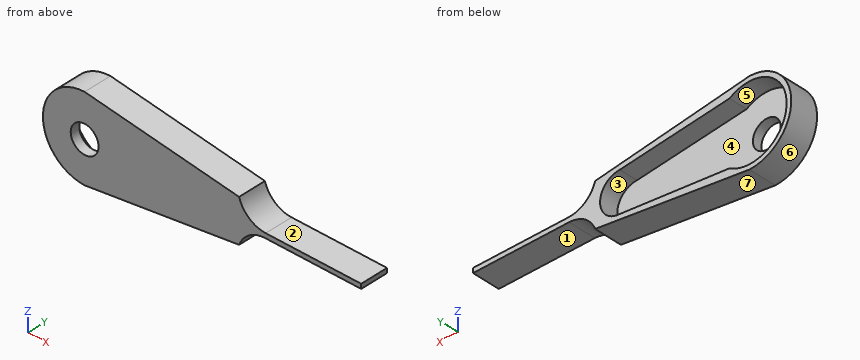
```python
from build123d import *

# Parameters (mm, degrees)
SKETCH2_R           = 1.5
BOSS_EXTRUDE1_DEPTH = 1
BOSS_EXTRUDE2_DEPTH = 3
FILLET1_R           = 3
FILLET2_R           = 3


with BuildPart() as part:
    # Sketch2 → Boss-Extrude1 (new body)
    with BuildSketch(Plane(origin=(0, 0, 0), x_dir=(1, 0, 0), z_dir=(0, 1, 0))):
        with BuildLine():
            Line((-12.939762178, 2.094266176), (-24.821781773, 3.29179515))
            ThreePointArc((-24.821781773, 3.29179515), (-30.987291256, -0.071668068), (-24.821747911, -3.435069212))
            Line((-24.821747911, -3.435069212), (-12.987160246, -2.166440487))
            ThreePointArc((-12.987160246, -2.166440487), (-10.8566751, -0.059524017), (-12.939762178, 2.094266176))
        make_face()
        with Locations(Location((-26.987114413, 0, 0), (0, 0, 270))):
            Circle(SKETCH2_R, mode=Mode.SUBTRACT)
    extrude(amount=BOSS_EXTRUDE1_DEPTH)

    # Sketch2<3> → Boss-Extrude2 (add)
    with BuildSketch(Plane(origin=(0, 0, 0), x_dir=(1, 0, 0), z_dir=(0, 1, 0))):
        with BuildLine():
            Line((-10.322349305, -2.339041202), (-10.322728968, -0.2))
            Line((-10.322728968, -0.2), (2.851540312, -0.2))
            Line((2.851540312, -0.2), (2.851540312, 0.3))
            Line((2.851540312, 0.3), (-10.322728968, 0.3))
            Line((-10.322728968, 0.3), (-10.322728968, 2.279037645))
            Line((-10.322728968, 2.279037645), (-26.987114411, 4.428185187))
            ThreePointArc((-26.987114411, 4.428185187), (-31.48694753, -0.071647931), (-26.987114411, -4.57148105))
            Line((-26.987114411, -4.57148105), (-10.322349305, -2.339041202))
        make_face()
        with BuildLine():
            ThreePointArc((-12.939762178, 2.094266176), (-10.8566751, -0.059524017), (-12.987160246, -2.166440487))
            Line((-12.987160246, -2.166440487), (-24.821747911, -3.435069212))
            ThreePointArc((-24.821747911, -3.435069212), (-30.987291256, -0.071668068), (-24.821781773, 3.29179515))
            Line((-24.821781773, 3.29179515), (-12.939762178, 2.094266176))
        make_face(mode=Mode.SUBTRACT)
    extrude(amount=BOSS_EXTRUDE2_DEPTH)

    # Fillet1
    # the kernel refuses this fillet: 3 mm, written as the material it adds along each edge
    with BuildSketch(Plane(origin=(-10.322728968, 0, -0.3), x_dir=(1, 0, 0), z_dir=(0, 1, 0))) as fillet1_piece_1:
        with BuildLine():
            CenterArc((2.820928193, 3), FILLET1_R, 199.896419226, 70.103580774)
            Line((0, 1.979037645), (-0.056418564, 1.958618398))
            ThreePointArc((-0.056418564, 1.958618398), (-0.06, 0.989518822), (-0.06, 0))
            Line((-0.06, 0), (0, -0.06))
            Line((0, -0.06), (2.820928193, -0.06))
            Line((2.820928193, -0.06), (2.820928193, 0))
        make_face()
    extrude(amount=3)

    # Fillet2
    # the kernel refuses this fillet: 3 mm, written as the material it adds along each edge
    with BuildSketch(Plane(origin=(-10.322728968, 0, 0.2), x_dir=(1, 0, 0), z_dir=(0, 1, 0))) as fillet2_piece_1:
        with BuildLine():
            CenterArc((2.874183753, -3), FILLET2_R, 90, 73.322386102)
            Line((0.000379663, -2.139041202), (-0.057096419, -2.121822026))
            ThreePointArc((-0.057096419, -2.121822026), (-0.059810168, -1.069531251), (-0.059999999, -1.065e-05))
            Line((-0.059999999, -1.065e-05), (0, 0.06))
            Line((0, 0.06), (2.874183753, 0.06))
            Line((2.874183753, 0.06), (2.874183753, 0))
        make_face()
    extrude(amount=3)


solid = part.part
```
Read the model definition and answer for the solid it produces. Units are mm, in the model's axes. Face numbers are marked on the shaded views. A direction names the side the tool comes from. Give positions to 0.01 mm unless a question says otherwise; leave off trailing zeros. Loops run counter-clockwise (first coordinate to the right, second up) from the corner with the lowest first, then second, coordinate; pieces in that order, holes last.
Item 1: Find the intervals of material crossed by line 1 along X through (y, z) = (0.6, 0); line 2 along Z through (x, y) = (-4.5, 0.4); line 3 along Y through (x, z) = (-15, 0.25), in increasing order.
Item 2: The mould has two halves that part along Z. Classify the marked faces 4, 5, 6 and 7: released by +Z, released by -Z, zero draft, split by the parting line, or undercut.
Item 3: The part is cut by section D-D (x = -2). Write down the section's boundary in (y, z), and give its area (3 significant figures).
Item 4: The part is cut by section B-B (x = -24.5). Write down the section's boundary in (y, z), and give its area (3 significant figures).
Item 5: The part is cut by section A-A (y = 0.35). Write down the section's boundary in (x, z).
Item 6: The part is cut by section C-C (y = 2.1). Write down the section's boundary in (x, z).
Item 7: For the marked faces 1, 2 and 3, determine the directions among +Z, -Z, +X, -X, +Y, -Y from which every point of the face is accessible in a straight line to the end or side of a thin tool.
Item 8: Each of these flat-tipped pins is pushed along its axis until it touches: pin 1 Ø1.5 at (x, y) = (-4, 1) entering from -Z; pin 2 Ø3.5 at (x, z) = (-26.99, 0) entering from +Y. Where does it stop, or does it pass through?
Taken from the geometry:
1. line 1: x = -31.49 to -28.49, -25.49 to 2.85
1. line 2: z = -0.3 to 0.2
1. line 3: y = 0 to 1
2. face 4: undercut
2. face 5: undercut
2. face 6: split by the parting line
2. face 7: released by -Z
3. outline: (0, -0.3) - (3, -0.3) - (3, 0.2) - (0, 0.2) - close
3. area: 1.50 mm2
4. outline: (0, -4.11) - (3, -4.11) - (3, -3.26) - (1, -3.26) - (1, 3.4) - (3, 3.4) - (3, 4.24) - (0, 4.24) - close
4. area: 11.7 mm2
5. outline: (-26.99, -4.43) - (-10.32, -2.28) arc R3 cw to (-7.5, -0.3) - (2.85, -0.3) - (2.85, 0.2) - (-7.45, 0.2) arc R3 cw to (-10.32, 2.34) - (-26.99, 4.57) arc R4.5 ccw to start; hole circle Ø3 at (-26.99, 0)
6. outline: (-26.99, -4.43) - (-10.32, -2.28) arc R3 cw to (-7.5, -0.3) - (2.85, -0.3) - (2.85, 0.2) - (-7.45, 0.2) arc R3 cw to (-10.32, 2.34) - (-26.99, 4.57) arc R4.5 ccw to start; hole (-24.82, -3.29) - (-12.94, -2.09) arc R2.13 ccw to (-12.99, 2.17) - (-24.82, 3.44) arc R4 ccw (long way) to start
7. face 1: -Z, +X, +Y, -Y
7. face 2: +Z, +X, +Y, -Y
7. face 3: +Y
8. pin 1: stops at z = -0.3
8. pin 2: stops at y = 1
